Drawing for the job (mm, zero at the part's lowest x, y, z). A direction names the side the tool comes from. Round coordinates to 2 decimals unless told otherwise and drop trailing zeros. Order: outer loops, then holes, each group sorted by start corner. A loop starts at its lowest first (then second) coordinate and runs counter-clockwise, first axis right, second up. Notation, with made-up numbers: (10, 27) - (69, 27) arc R7 ccw to (69, 39) - close; hole circle Ø9 at (24.25, 17.5). An arc over 180 degrees is marked (long way). Put each result on its own line as item: value. Start each with the question number.
Item 1: Saw through at C-C on z = 75. List the corners of the cut face in (x, y).
Item 2: Mould opens along Y. For the marked faces 3, 4 and 5 say: pulls with the +Y half, pulls with the -Y half, needs draft (parallel to the pull), parting line crosses it, or undercut.
Item 3: Saw through at D-D on x = 13.5. List the corners of the cut face in (y, z).
Item 4: Saw through at A-A on y = 55. List the corners of the cut face in (x, z), plus the area to 3 significant figures.
Item 5: Which spindle directions (+Z, -Z, +X, -X, +Y, -Y) get a long thin tool onto all of the face, cutting with end or side? Do the marked faces 1 and 2. Say none if no direction does.
Item 6: Probe probe 1 along Y at (x, z) = (10.75, 50); probe 2 along Z at (x, y) = (4.5, 7) (1 decimal); probe 3 along Z at (x, y) = (1.25, 125.5). List the from-to ranges inside material, lowest first.
Item 7: Saw through at B-B on y = 7.5. List the corners of the cut face in (x, z).
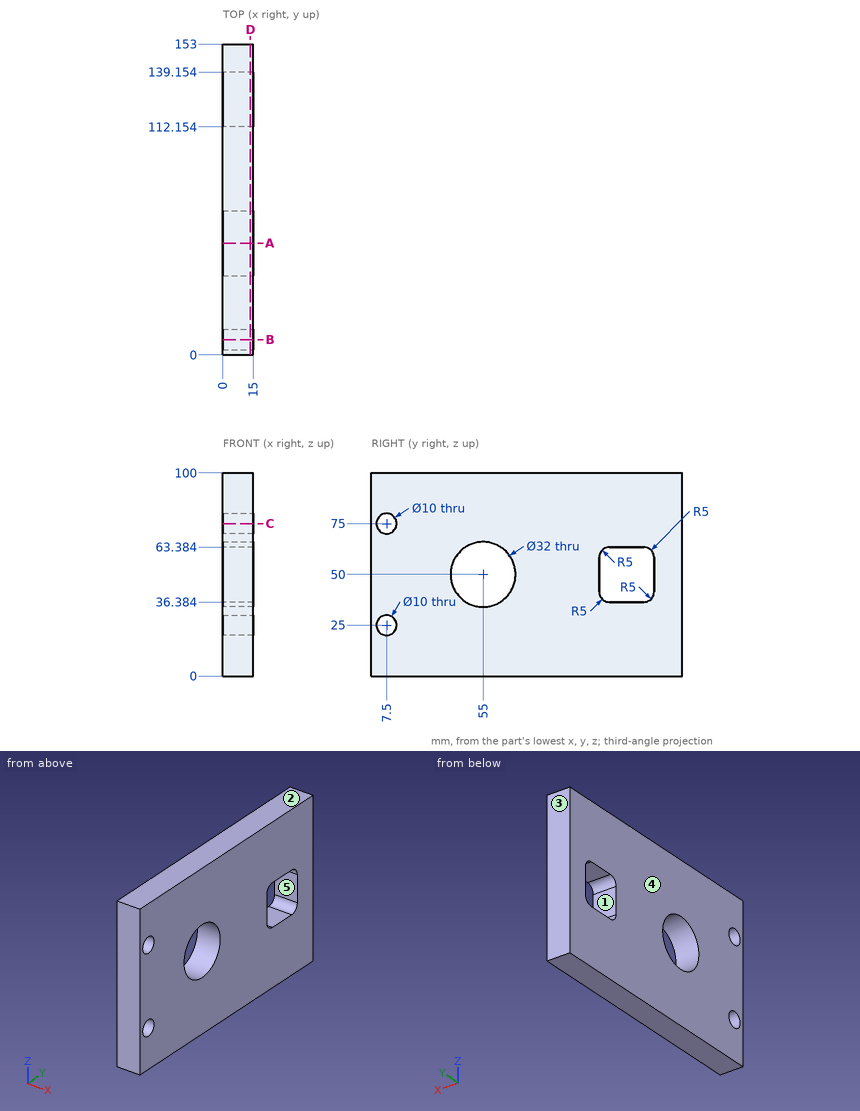
Results found:
1. outline: (0, 0) - (15, 0) - (15, 2.5) - (0, 2.5) - close; (0, 12.5) - (15, 12.5) - (15, 153) - (0, 153) - close
2. face 3: pulls with the +Y half
2. face 4: needs draft
2. face 5: undercut
3. outline: (0, 0) - (153, 0) - (153, 100) - (0, 100) - close; hole circle Ø10 at (7.5, 25); hole circle Ø10 at (7.5, 75); hole circle Ø32 at (55, 50); hole (112.15, 41.38) arc R5 ccw to (117.15, 36.38) - (134.15, 36.38) arc R5 ccw to (139.15, 41.38) - (139.15, 58.38) arc R5 ccw to (134.15, 63.38) - (117.15, 63.38) arc R5 ccw to (112.15, 58.38) - close
4. outline: (0, 0) - (15, 0) - (15, 34) - (0, 34) - close; (0, 66) - (15, 66) - (15, 100) - (0, 100) - close
4. area: 1,020 mm²
5. face 1: +X, -X
5. face 2: +Z, +X, -X, +Y, -Y
6. probe 1: y = 0 to 39, 71 to 112.15, 139.15 to 153
6. probe 2: z = 0 to 20, 30 to 70, 80 to 100
6. probe 3: z = 0 to 36.38, 63.38 to 100
7. outline: (0, 0) - (15, 0) - (15, 20) - (0, 20) - close; (0, 30) - (15, 30) - (15, 70) - (0, 70) - close; (0, 80) - (15, 80) - (15, 100) - (0, 100) - close
